```python
from build123d import *

# Parameters (mm, degrees)
BOSS_EXTRU_2_DEPTH      = 20
ESQUISSE3_R             = 1.75
ENL_V_MAT_EXTRU_2_DEPTH = 4
ESQUISSE4_R             = 3.5
ENL_V_MAT_EXTRU_3_DEPTH = 13


with BuildPart() as part:
    # Esquisse1 → Boss.-Extru.2 (new body)
    with BuildSketch(Plane.XY):
        with BuildLine():
            Line((-20, 0.5), (-16.124515497, 0.5))
            ThreePointArc((-16.124515497, 0.5), (-14.241577753, 1.164503168), (-13.192785406, 2.863636364))
            ThreePointArc((-13.192785406, 2.863636364), (0, 13.5), (13.192785406, 2.863636364))
            ThreePointArc((13.192785406, 2.863636364), (14.241577753, 1.164503168), (16.124515497, 0.5))
            Line((16.124515497, 0.5), (20, 0.5))
            Line((20, 0.5), (20, 3.5))
            Line((20, 3.5), (15.099668871, 3.5))
            ThreePointArc((15.099668871, 3.5), (0, 15.5), (-15.099668871, 3.5))
            Line((-15.099668871, 3.5), (-20, 3.5))
            Line((-20, 3.5), (-20, 0.5))
        make_face()
    extrude(amount=BOSS_EXTRU_2_DEPTH)

    # Esquisse3 → Enlèv. mat.-Extru.2 (cut, through all)
    with BuildSketch(Plane(origin=(0, 3.5, 0), x_dir=(1, 0, 0), z_dir=(0, 1, 0))):
        with Locations((-17, -10)):
            Circle(ESQUISSE3_R)
        with Locations((17, -10)):
            Circle(ESQUISSE3_R)
    extrude(amount=-ENL_V_MAT_EXTRU_2_DEPTH, mode=Mode.SUBTRACT)

    # Esquisse4 → Enlèv. mat.-Extru.3 (cut, through all)
    with BuildSketch(Plane(origin=(0, 3.5, 0), x_dir=(1, 0, 0), z_dir=(0, 1, 0))):
        with Locations((-17, -10)):
            Circle(ESQUISSE4_R)
        with Locations((17, -10)):
            Circle(ESQUISSE4_R)
    extrude(amount=ENL_V_MAT_EXTRU_3_DEPTH, mode=Mode.SUBTRACT)


solid = part.part
```
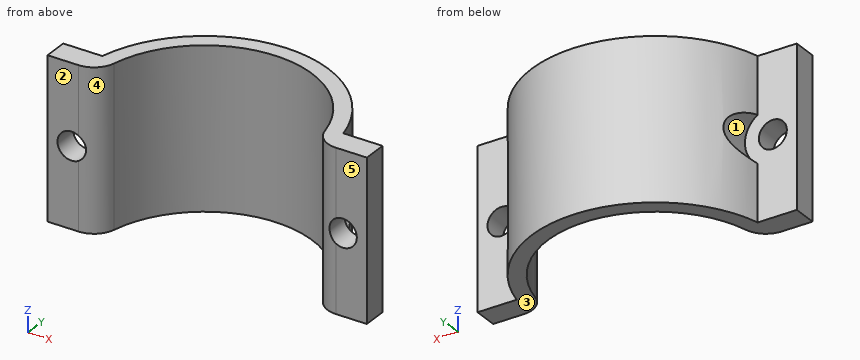
Source: CAD feature listing. Evaluate the final solid. Frame: model axes, mm. Face numbers are marked on the shaded views. A direction names the side the tool comes from. Give positions to 0.01 mm unless a question says otherwise; leave off trailing zeros. Loops run counter-clockwise (first coordinate to the right, second up) from the corner with the lowest first, then second, coordinate; pieces in that order, holes last. Notation, with made-up numbers: (38, -20) -> (58, -20) arc R25 ccw to (58, -7) -> close; hole circle Ø2 at (46.5, 18). An arc over 180 degrees is marked (long way). Use a Markdown table: item, result. Add a question column.
(1) Pull-direction query (Z, two-part tool) for the marked faces 1, 2 and 3; classes: +Z half, -Z half, draft (parallel to the pull), parting line (faces both ways), or undercut.
(2) Access query for the marked faces 4 and 5. Directions: +Z, -Z, +X, -X, +Y, -Y. A direction counts if a zero-diameter tool reaches every point of the face in a straight line with its end or side. Return the directions, or none.
(3) First-contact query: pin 1 Ø6 at (y, z) = (8, 14) entering from -X; pin 2 Ø4 at (x, z) = (-11.5, 10) entering from -Y; pin 3 Ø8 at (x, z) = (2.5, 10) entering from -Y. Flat tips, straight axial feed; report the tip coordinate or a pass-through.
(4) Section query D-D (z = 10). Output: boundary loops of the cut face in (x, y), then the cut area to 3 significant figures.
(5) Section query C-C (z = 15). Output: boundary loops of the cut face in (x, y), then the cut area to 3 significant figures.
(6) Section query A-A (x = -17). Output: boundary loops of the cut face in (y, z), then the cut area to 3 significant figures.
(7) Section query B-B (y = 2.25). Output: boundary loops of the cut face in (x, z), then the cut area to 3 significant figures.
(8) Ray query, line 1 (X direction, y = 2.15, z = 10); line 2 (X direction, y = 1.5, z = 10); line 3 (Z direction, x = 17, y = 2.8). Return the intervals inside material, ascending.
Checked values:
| question | item | result |
|---|---|---|
| 1 | face 1 | undercut |
| 1 | face 2 | draft |
| 1 | face 3 | -Z half |
| 2 | face 4 | +Z, -Z, -Y |
| 2 | face 5 | +Z, -Z, +X, -X, -Y |
| 3 | pin 1 | x = -14.67 |
| 3 | pin 2 | y = 2.05 |
| 3 | pin 3 | y = 11.83 |
| 4 | outline | (-20, 0.5) -> (-18.75, 0.5) -> (-18.75, 3.5) -> (-20, 3.5) -> close; (-15.25, 0.63) arc R3 ccw to (-13.19, 2.86) arc R13.5 cw to (13.19, 2.86) arc R3 ccw to (15.25, 0.63) -> (15.25, 3.5) -> (13.5, 3.5) -> (13.5, 7.62) arc R15.5 ccw to (-13.5, 7.62) -> (-13.5, 3.5) -> (-15.25, 3.5) -> close; (18.75, 0.5) -> (20, 0.5) -> (20, 3.5) -> (18.75, 3.5) -> close |
| 4 | area | 86.0 mm^2 |
| 5 | outline | (-20, 0.5) -> (-16.12, 0.5) arc R3 ccw to (-13.19, 2.86) arc R13.5 cw to (13.19, 2.86) arc R3 ccw to (16.12, 0.5) -> (20, 0.5) -> (20, 3.5) -> (15.1, 3.5) arc R15.5 ccw to (-15.1, 3.5) -> (-20, 3.5) -> close |
| 5 | area | 114 mm^2 |
| 6 | outline | (0.5, 0) -> (3.5, 0) -> (3.5, 8.25) -> (0.5, 8.25) -> close; (0.5, 11.75) -> (3.5, 11.75) -> (3.5, 20) -> (0.5, 20) -> close |
| 6 | area | 49.5 mm^2 |
| 7 | outline | (-20, 0) -> (-13.4, 0) -> (-13.4, 20) -> (-20, 20) -> close; (13.4, 0) -> (20, 0) -> (20, 20) -> (13.4, 20) -> close; hole circle Ø3.5 at (-17, 10); hole circle Ø3.5 at (17, 10) |
| 7 | area | 245 mm^2 |
| 8 | line 1 | -20 to -18.75, -15.25 to -13.45, 13.45 to 15.25, 18.75 to 20 |
| 8 | line 2 | -20 to -18.75, -15.25 to -13.89, 13.89 to 15.25, 18.75 to 20 |
| 8 | line 3 | 0 to 8.25, 11.75 to 20 |
